Design review of the part built by this model. Coordinates are the model's own, in mm. Face numbers are marked on the shaded views. Coordinates: 2 decimals unless noted, no trailing zeros. Loops run counter-clockwise (first coordinate to the right, second up) from the corner with the lowest first, then second, coordinate; pieces in that order, holes last.
Q1. Draft analysis for pull direction X (two halves, no side actions). For the marked faces 1, 2 and 3, state which applies: released by +X, released by -X, zero draft, split by the parting line, or undercut.
Q2. Add section A-A on y = -30. Give the boundary of the cut face in (x, z), and give its area (3 significant figures).
Q3. Wall thickness on probe 1 along Z at (x, y) = (-57.5, -39.5); probe 2 along X at (y, z) = (-53, 31.5): over which ranges is each line inside the solid? List them lowest first.
Q4. For P1, Ø2.5, axis at x = -68, z = -38.5, coming from the +Y side; P2, Ø1.5, axis at x = -68.5, z = -37.5, coming from the -Y side, all flat-tipped, find the tip position at first contact; note any pin that passes through.
Q5. Add section C-C on z = -25.5. Give the boundary of the cut face in (x, y), and give its area (3 significant figures).
Q6. Add section B-B on x = -56.5. Give the boundary of the cut face in (y, z), and give its area (3 significant figures).
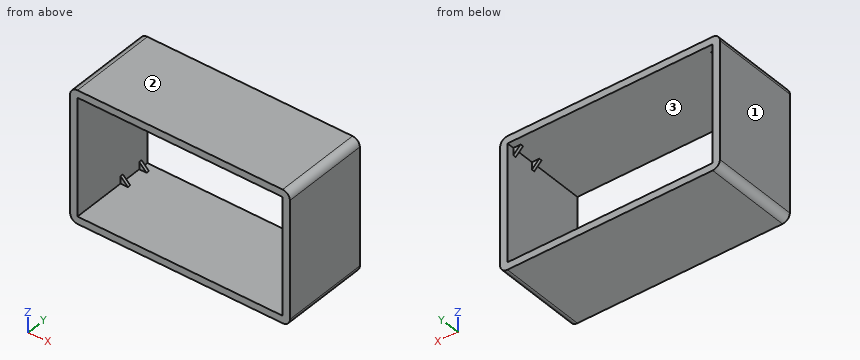
```python
from build123d import *

# Parameters (mm, degrees)
F0_W     = 1500
F0_H     = 900
F0_W_2   = 1400
F0_H_2   = 800
F1_DEPTH = 600
F2_SCALE = 0.1
F6_DEPTH = 2
F7_R     = 5


# Not quite as in the source:
# - a pattern or mirror of a feature is missing from the dataset's text; its kind, count and spacing are read off the source's solid


with BuildPart() as f1:
    # F0 (on Front) → F1 (new body)
    with BuildSketch(Plane.XZ):
        Rectangle(F0_W, F0_H)
        Rectangle(F0_W_2, F0_H_2, mode=Mode.SUBTRACT)
    extrude(amount=F1_DEPTH)


with BuildPart() as f1_1:
    # F2: moved
    add(f1.part.scale(F2_SCALE))

    # F5 (on offset) → F6 (join)
    with BuildSketch(Plane(origin=(0, -21, 0), x_dir=(-1, 0, 0), z_dir=(0, 1, 0))):
        Polygon((-65, 40), (-70, 40), (-70, 35), align=None)
        Polygon((65, 40), (70, 35), (70, 40), align=None)
        Polygon((-70, -35), (-70, -40), (-65, -40), align=None)
        Polygon((65, -40), (70, -40), (70, -35), align=None)
    f6 = extrude(amount=-F6_DEPTH)

    # F6_copies: F6 across plane
    add(f6.mirror(Plane.ZX.offset(-14)))

    # F7
    f7_edges = [f1_1.edges().sort_by_distance(p)[0] for p in [
        (75, -30, 45),
        (75, -30, -45),
        (-75, -30, -45),
        (-75, -30, 45),
    ]]
    fillet(f7_edges, radius=F7_R)


solid = f1_1.part
```
Entries:
1. face 1: released by -X
1. face 2: zero draft
1. face 3: undercut
2. outline: (-75, -40) arc R5 ccw to (-70, -45) - (70, -45) arc R5 ccw to (75, -40) - (75, 40) arc R5 ccw to (70, 45) - (-70, 45) arc R5 ccw to (-75, 40) - close; hole (-70, -40) - (70, -40) - (70, 40) - (-70, 40) - close
2. area: 2,280 mm2
3. probe 1: z = -45 to -40, 40 to 45
3. probe 2: x = -75 to -70, 70 to 75
4. P1: stops at y = -5
4. P2: stops at y = -23
5. outline: (-75, -60) - (-70, -60) - (-70, 0) - (-75, 0) - close; (70, -60) - (75, -60) - (75, 0) - (70, 0) - close
5. area: 600 mm2
6. outline: (-60, -45) - (0, -45) - (0, -40) - (-60, -40) - close; (-60, 40) - (0, 40) - (0, 45) - (-60, 45) - close
6. area: 600 mm2
